```python
from build123d import *

# Parameters (mm, degrees)
SKETCH1_W                   = 19.05
SKETCH1_H                   = 63.5
BOSS_EXTRUDE1_DEPTH         = 63.5
F_1_4_20_TAPPED_HOLE1_D     = 5.1054
F_1_4_20_TAPPED_HOLE1_DEPTH = 16.51
F_1_4_20_TAPPED_HOLE1_TIP   = 1.533816902
F_1_4_20_TAPPED_HOLE2_D     = 5.1054
F_1_4_20_TAPPED_HOLE2_DEPTH = 16.51
F_1_4_20_TAPPED_HOLE2_TIP   = 1.533816902


with BuildPart() as part:
    # Sketch1 → Boss-Extrude1 (new body)
    with BuildSketch(Plane(origin=(0, 0, 0), x_dir=(1, 0, 0), z_dir=(0, 1, 0))):
        Rectangle(SKETCH1_W, SKETCH1_H)
    extrude(amount=BOSS_EXTRUDE1_DEPTH)

    # 1/4-20 Tapped Hole1
    with Locations(Plane(origin=(0, 0, 0), x_dir=(-1, 0, 0), z_dir=(0, -1, 0))):
        with Locations((0, -25.4), (0, 25.4)):
            Hole(F_1_4_20_TAPPED_HOLE1_D / 2, depth=F_1_4_20_TAPPED_HOLE1_DEPTH)
            with Locations((0, 0, -(F_1_4_20_TAPPED_HOLE1_DEPTH + F_1_4_20_TAPPED_HOLE1_TIP / 2))):  # 118° drill point
                Cone(0, F_1_4_20_TAPPED_HOLE1_D / 2, F_1_4_20_TAPPED_HOLE1_TIP, mode=Mode.SUBTRACT)

    # 1/4-20 Tapped Hole2
    with Locations(Plane(origin=(0, 63.5, 0), x_dir=(1, 0, 0), z_dir=(0, 1, 0))):
        with Locations((0, 25.4), (0, -25.4)):
            Hole(F_1_4_20_TAPPED_HOLE2_D / 2, depth=F_1_4_20_TAPPED_HOLE2_DEPTH)
            with Locations((0, 0, -(F_1_4_20_TAPPED_HOLE2_DEPTH + F_1_4_20_TAPPED_HOLE2_TIP / 2))):  # 118° drill point
                Cone(0, F_1_4_20_TAPPED_HOLE2_D / 2, F_1_4_20_TAPPED_HOLE2_TIP, mode=Mode.SUBTRACT)


solid = part.part
```
For this review, take the finished solid that the model builds, in its own axes (mm). A direction names the side the tool comes from. Coordinates: 2 decimals unless noted, no trailing zeros. Loops run counter-clockwise (first coordinate to the right, second up) from the corner with the lowest first, then second, coordinate; pieces in that order, holes last.
1. Mouldability with a two-part tool opening along X and no side actions: class faces 1 (the flat face through (0, 31, -31.75)), 2 (the conical face through (-0.058, 45.723, -25.84)), 3 (the cylindrical face through (1.372, 8.371, -27.552)), 4 (the flat face through (9.525, 31, 0)) as +X half, -X half, draft (parallel to the pull), parting line (faces both ways), or undercut.
2. For line 1 (Z direction, x = 0, y = 5.25); line 2 (X direction, y = 53.5, z = 25.4) (3 decimals); line 3 (Z direction, x = -1.25, y = 16.5), list the stretches that pass through material, from the lowest coordinate up.
3. Insertion check: P1, Ø6, axis at x = 0, z = -25.4, coming from the -Y side; P2, Ø3, axis at x = 0, z = 25.4, coming from the -Y side. Each pin has a flat end and moves straight along its axis. Give the tip position at first contact, or say it passes through.
4. For faces 5 (the flat face through (0, 0, 0)), 6 (the cylindrical face through (2.03, 55.13, 26.95)), 7 (the cylindrical face through (-2.03, 8.37, 26.95)), list the 3-axis set-ups (+Z, -Z, +X, -X, +Y, -Y) from which the entire face can be reached by the end or side of a thin tool; tool diameter is ignored.
5. Add section A-A, the plane y = 5.5. Give the boundary of the cut face in (x, z) (3 decimals).
Result:
1. face 1: draft
1. face 2: undercut
1. face 3: undercut
1. face 4: +X half
2. line 1: z = -31.75 to -27.95, -22.85 to 22.85, 27.95 to 31.75
2. line 2: x = -9.525 to -2.553, 2.553 to 9.525
2. line 3: z = -31.75 to -27.63, -23.17 to 23.17, 27.63 to 31.75
3. P1: stops at y = 0
3. P2: stops at y = 17.14
4. face 5: +Z, -Z, +X, -X, -Y
4. face 6: +Y
4. face 7: -Y
5. outline: (-9.525, -31.75) - (9.525, -31.75) - (9.525, 31.75) - (-9.525, 31.75) - close; hole circle Ø5.105 at (0, -25.4); hole circle Ø5.105 at (0, 25.4)
